Answer from the drawing. Dimensions are ordinates in mm from the lowest x, y and z of the part. A direction names the side the tool comes from. Round coordinates to 2 decimals unless told otherwise and drop trailing zeros. Write each loop counter-clockwise with the first axis right and the second up, starting at its lowest first coordinate (ties: lowest second). Pieces come first, ordered by that corner, then holes. Notation, with made-up numbers: (64.5, 11) -> (103.5, 11) arc R22 cw to (103.5, 24) -> close; hole circle Ø9 at (70, 73). An arc over 180 degrees is marked (long way). Answer as a JSON object with one key per item and string values. Group by question number.
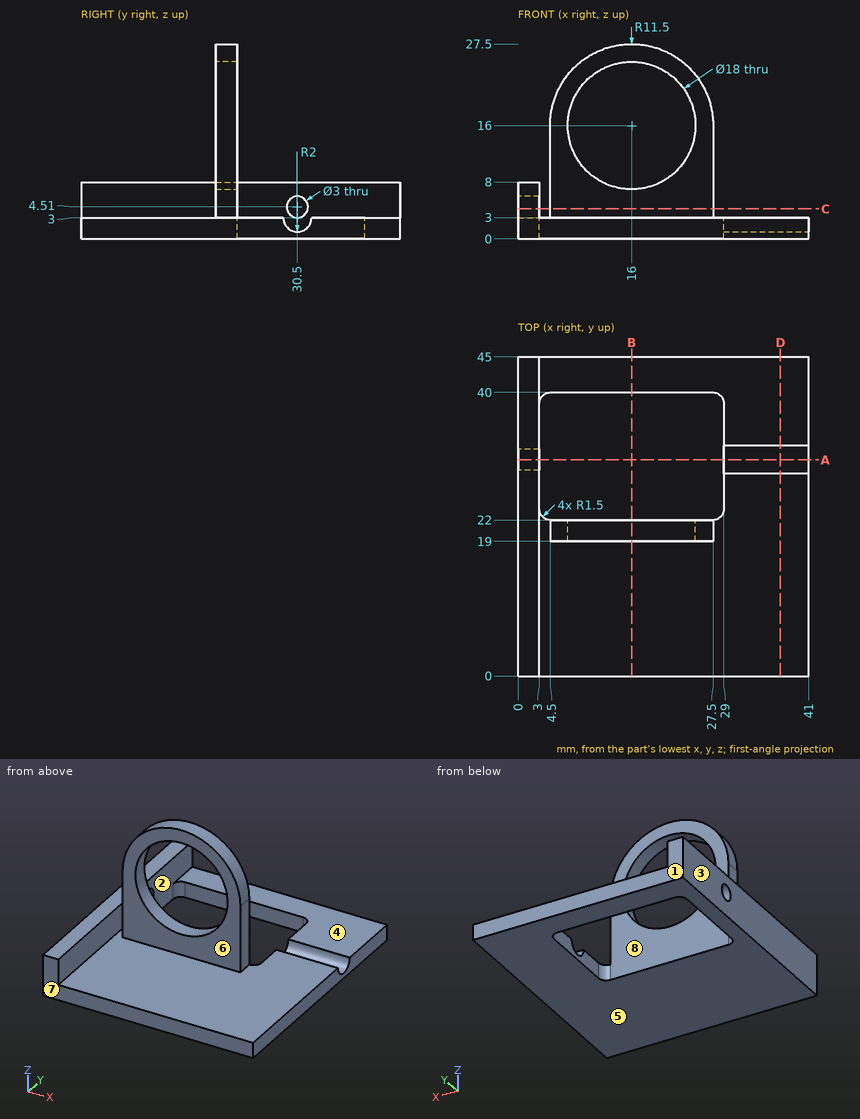
1) Straight lines are drawn through the part: L1, parallel to X at y = 20.75, z = 16; L2, parallel to Y at x = 21, z = 1.5; L3, parallel to Y at x = 2.2, z = 4.51. For each, find the intervals that lie inside material, in ascending order.
2) For a pull along X with two mould halves and no side action, classify the marked faces 1, 2 and 3 as released by +X, released by -X, zero draft, split by the parting line, or undercut.
3) A cutting plane is placed at B-B on x = 16. Determine the outline of the cut face in (y, z), plus the area to 4 significant figures.
4) A cutting plane is placed at A-A on y = 30.5. Determine the outline of the cut face in (x, z), plus the area to 3 significant figures.
5) A tool of negligible diameter and unlimited length cuts with its end or side. For the marked faces 4, 5, 6, 7 and 8, from which of +Z, -Z, +X, -X, +Y, -Y can it reach the whole face along a straight path? Write none if from no direction.
6) A cutting plane is placed at D-D on x = 37. Determine the outline of the cut face in (y, z).
7) A cutting plane is placed at C-C on z = 4.25. Determine the outline of the cut face in (x, y).
8) Each of these flat-tipped pins is pushed along its axis until it touches: P1, Ø3, axis at y = 27, z = 5.5, coming from the +X side; P2, Ø12, axis at x = 19.5, z = 15, coming from the +Y side; P3, Ø0.9, axis at y = 20.5, z = 6.5, coming from the +X side; P4, Ø14.5, axis at x = 16, z = 16, coming from the -Y side. Where does it stop, or does it pass through?
Established:
{
 "1": {"L1": "x = 4.5 to 7, 25 to 27.5", "L2": "y = 0 to 22, 40 to 45", "L3": "y = 0 to 29, 32 to 45"},
 "2": {"face 1": "zero draft", "face 2": "undercut", "face 3": "released by -X"},
 "3": {"outline": "(0, 0) -> (22, 0) -> (22, 7) -> (19, 7) -> (19, 3) -> (0, 3) -> close; (19, 25) -> (22, 25) -> (22, 27.5) -> (19, 27.5) -> close; (40, 0) -> (45, 0) -> (45, 3) -> (40, 3) -> close", "area": "100.5 mm²"},
 "4": {"outline": "(0, 0) -> (3, 0) -> (3, 3.01) -> (0, 3.01) -> close; (0, 6.01) -> (3, 6.01) -> (3, 8) -> (0, 8) -> close; (29, 0) -> (41, 0) -> (41, 1) -> (29, 1) -> close", "area": "27.0 mm²"},
 "5": {"face 4": "+Z, +X, +Y", "face 5": "-Z, +X, -X, +Y, -Y", "face 6": "+Z, +X, -Y", "face 7": "+Z, -Z, +X, -X, -Y", "face 8": "+Z, -Z"},
 "6": {"outline": "(0, 0) -> (45, 0) -> (45, 3) -> (32.5, 3) arc R2 cw to (28.5, 3) -> (0, 3) -> close"},
 "7": {"outline": "(0, 0) -> (3, 0) -> (3, 29.02) -> (0, 29.02) -> close; (0, 31.98) -> (3, 31.98) -> (3, 45) -> (0, 45) -> close; (4.5, 19) -> (27.5, 19) -> (27.5, 22) -> (4.5, 22) -> close"},
 "8": {"P1": "stops at x = 3", "P2": "stops at y = 22", "P3": "stops at x = 27.5", "P4": "passes through"}
}
